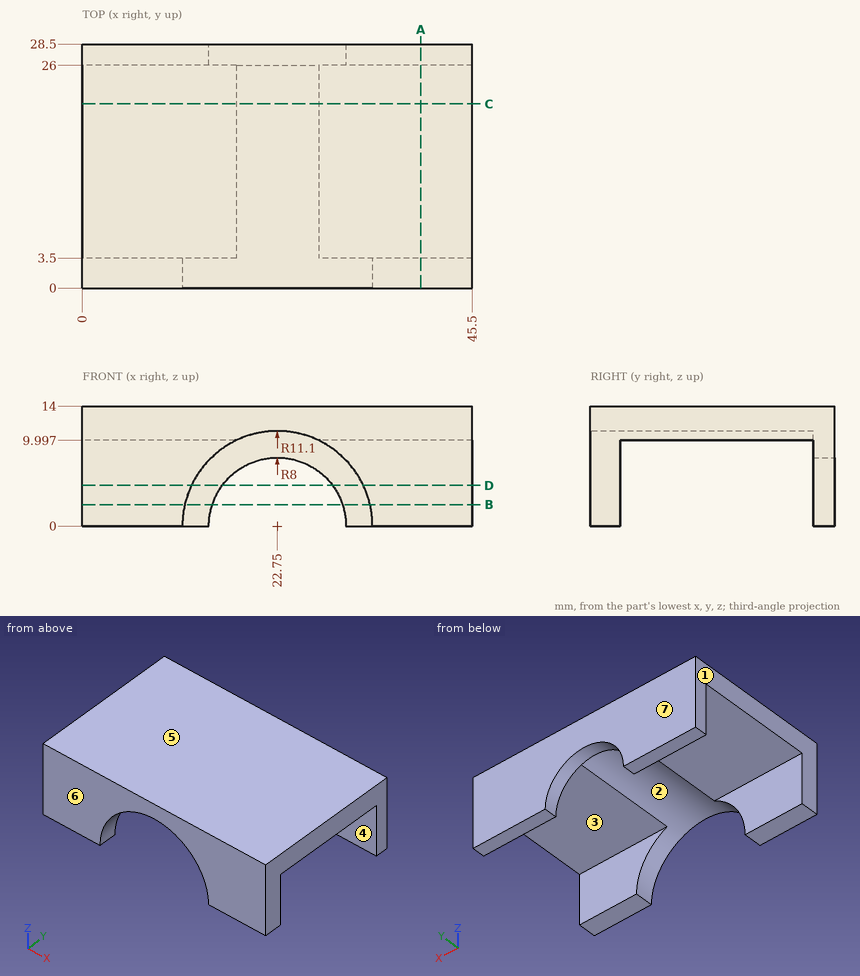
Can you work these out from the drawing? Everything is in mm from the part's minimum corner. A direction names the side the tool comes from. Coordinates: 2 decimals unless noted, no trailing zeros. Loops run counter-clockwise (first coordinate to the right, second up) from the corner with the lowest first, then second, coordinate; pieces in that order, holes last. Notation, with made-up numbers: (-38.5, 41.5) - (17.5, 41.5) arc R12 ccw to (17.5, 53.5) - close; hole circle Ø11 at (44.5, 77). An arc over 180 degrees is marked (long way). Put each result on its own line as item: value. Start each with the question number.
Item 1: If we mould it in two halves opening along Y, with no side actions, what happens to the marked faces 4, 5, 6 and 7? For each: +Y half, -Y half, draft (parallel to the pull), parting line (faces both ways), or undercut.
Item 2: Suppose I cut it at D-D (z = 4.75). Please give me the cut outline in (x, y), and give its area (3 significant figures).
Item 3: For pin 1 (4 mm diameter, centred on x = 12, z = 6.5, fed in from -Y); pin 2 (5.5 mm diameter, centred on x = 7.5, y = 17.5, fed in from -Z); pin 3 (8 mm diameter, centred on x = 27.5, y = 5.5, fed in from -Z) (1 decimal), each with a flat end and sliding along its axis, tell me the tip position at first contact or that it passes through.
Item 4: Suppose I cut it at B-B (z = 2.5). Please give me the cut outline in (x, y) (1 decimal).
Item 5: Suppose I cut it at C-C (y = 21.5). Please give me the cut outline in (x, z), and give its area (3 significant figures).
Item 6: Suppose I cut it at A-A (x = 39.5). Please give me the cut outline in (y, z).
Item 7: If I drill on line 1 along Y through (x, z) = (7, 4); line 2 along Z through (x, y) = (29, 4.5); line 3 along Z through (x, y) = (22, 14.5) (1 decimal), over which ranges is the centre line in solid material (lowest first)?
Item 8: Which directions (+Z, -Z, +X, -X, +Y, -Y) give clear straight access to the entire face, cutting with the end or side of a thin tool? Please do the marked faces 1, 2 and 3.
Here are the results:
1. face 4: undercut
1. face 5: draft
1. face 6: -Y half
1. face 7: +Y half
2. outline: (0, 0) - (12.72, 0) - (12.72, 3.5) - (0, 3.5) - close; (0, 26) - (16.31, 26) - (16.31, 28.5) - (0, 28.5) - close; (29.19, 26) - (45.5, 26) - (45.5, 28.5) - (29.19, 28.5) - close; (32.78, 0) - (45.5, 0) - (45.5, 3.5) - (32.78, 3.5) - close
2. area: 171 mm²
3. pin 1: y = 0
3. pin 2: z = 10
3. pin 3: z = 7.5
4. outline: (0, 0) - (11.9, 0) - (11.9, 3.5) - (0, 3.5) - close; (0, 26) - (15.2, 26) - (15.2, 28.5) - (0, 28.5) - close; (30.3, 26) - (45.5, 26) - (45.5, 28.5) - (30.3, 28.5) - close; (33.6, 0) - (45.5, 0) - (45.5, 3.5) - (33.6, 3.5) - close
5. outline: (0, 10) - (17.93, 10) arc R11.1 cw to (27.57, 10) - (45.5, 10) - (45.5, 14) - (0, 14) - close
5. area: 175 mm²
6. outline: (0, 0) - (3.5, 0) - (3.5, 10) - (26, 10) - (26, 0) - (28.5, 0) - (28.5, 14) - (0, 14) - close
7. line 1: 0 to 3.5, 26 to 28.5
7. line 2: 10 to 14
7. line 3: 11.1 to 14
8. face 1: +Z, -Z, -X, +Y, -Y
8. face 2: -Z, -Y
8. face 3: -Z, +X, -X
